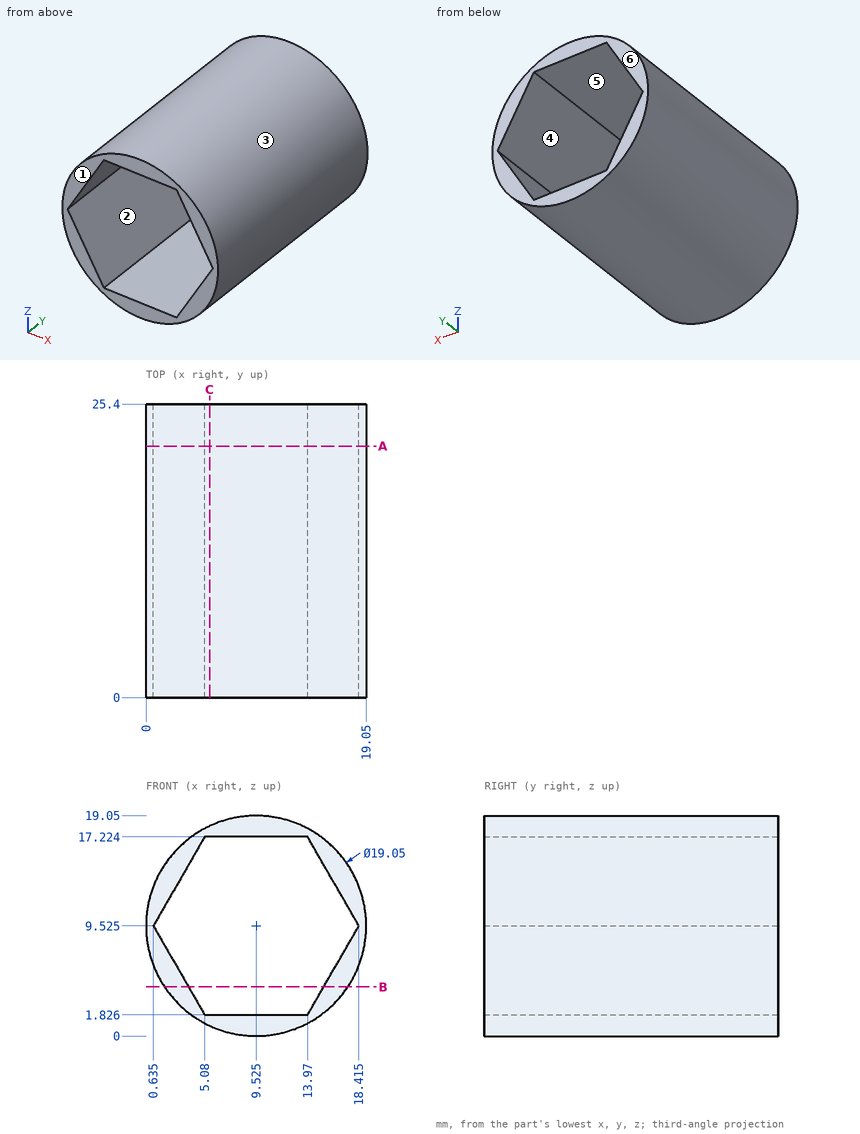
Design review of the part shown in the three views and the two pictorial views. Dimensions are in mm from the part's minimum x, y and z. A direction names the side the tool comes from. Round coordinates to 2 decimals unless told otherwise and drop trailing zeros. Loops run counter-clockwise (first coordinate to the right, second up) from the corner with the lowest first, then second, coordinate; pieces in that order, holes last. Notation, with made-up numbers: M 43,82.5 L 78,82.5 A28 ccw 78,104.5 Z; hole C 25.25,-24 d5. An arc over 180 degrees is marked long. Answer as a JSON object with one key per item and string values.
Item 1: We need section C-C, the plane x = 5.5. State the section outline as (y, z) points, and give its area (3 significant figures).
Check sheet entries:
{"outline": "M 0,0.89 L 25.4,0.89 L 25.4,1.83 L 0,1.83 Z; M 0,17.22 L 25.4,17.22 L 25.4,18.16 L 0,18.16 Z", "area": "47.4 mm2"}
Item 2: We need section B-B, the plane z = 4.25. State the section outline as (x, y) points.
Check sheet entries:
{"outline": "M 1.59,0 L 3.68,0 L 3.68,25.4 L 1.59,25.4 Z; M 15.37,0 L 17.46,0 L 17.46,25.4 L 15.37,25.4 Z"}
Item 3: Clearance check with flat-ended pins moving along their axes: P1, Ø5, axis at x = 5.5, y = 5.5, coming from the -Z side; P2, Ø1.5, axis at x = 14, y = 12.5, coming from the +Z side; P3, Ø3, axis at y = 14.5, z = 13, coming from the -X side. State where each tip first meets the part, or that it passes through.
Check sheet entries:
{"P1": "z = 0.12", "P2": "z = 18.29", "P3": "x = 0.21"}
Item 4: The part is to be moulded in two halves that separate along X. For the marked faces 1, 2, 3 and 4, say which applies: +X half, -X half, draft (parallel to the pull), parting line (faces both ways), or undercut.
Check sheet entries:
{"face 1": "draft", "face 2": "undercut", "face 3": "parting line", "face 4": "undercut"}
Item 5: We need section A-A, the plane y = 21.75. State the section outline as (x, z) points (3 decimals).
Check sheet entries:
{"outline": "C 9.525,9.525 d19.05; hole M 0.635,9.525 L 5.08,1.826 L 13.97,1.826 L 18.415,9.525 L 13.97,17.224 L 5.08,17.224 Z"}
Item 6: Tool access review of the marked faces 5 and 6: name each direction out of +Z, -Z, +X, -X, +Y, -Y from which nothing blocks a thin tool from reaching the whole face with its end or side.
Check sheet entries:
{"face 5": "+Y, -Y", "face 6": "+Z, -Z, +X, -X, +Y"}
Item 7: For line 1 along Z through (x, y) = (10.75, 18); line 2 along X through (y, z) = (15, 13.75); line 3 along X through (y, z) = (12.5, 9), list the stretches that pass through material, from the lowest coordinate up.
Check sheet entries:
{"line 1": "0.08 to 1.83, 17.22 to 18.97", "line 2": "0.99 to 3.07, 15.98 to 18.06", "line 3": "0.01 to 0.94, 18.11 to 19.04"}
